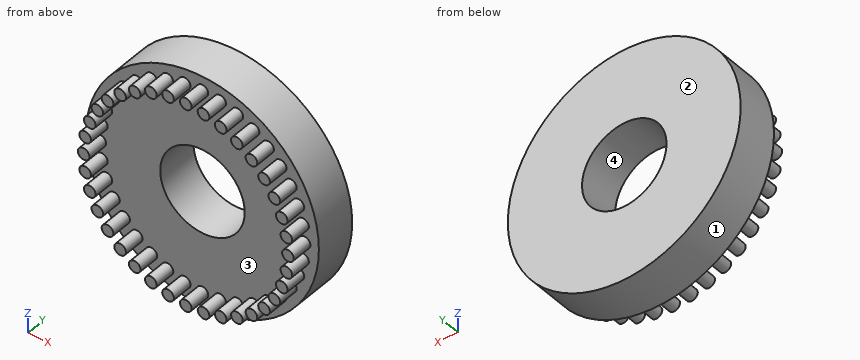
```python
from build123d import *

# Parameters (mm, degrees)
F0_R     = 35
F1_DEPTH = 12.7
F2_R     = 1.75
F3_DEPTH = 6.35
F4_R     = 12.7
F5_DEPTH = 12.701


with BuildPart() as f1:
    # F0 (on Front) → F1 (new body)
    with BuildSketch(Plane.XZ):
        Circle(F0_R)
    extrude(amount=F1_DEPTH)

    # F2 (on face) → F3 (join)
    with BuildSketch(Plane.XZ.offset(12.7)):
        with Locations((-30.708063, 0)):
            Circle(F2_R)
        with Locations((-30.241539, 5.332399)):
            Circle(F2_R)
        with Locations((-28.856141, 10.502776)):
            Circle(F2_R)
        with Locations((-26.593963, 15.354032)):
            Circle(F2_R)
        with Locations((-23.523741, 19.738763)):
            Circle(F2_R)
        with Locations((-19.738763, 23.523741)):
            Circle(F2_R)
        with Locations((-15.354032, 26.593963)):
            Circle(F2_R)
        with Locations((-10.502776, 28.856141)):
            Circle(F2_R)
        with Locations((-5.332399, 30.241539)):
            Circle(F2_R)
        with Locations((0, 30.708063)):
            Circle(F2_R)
        with Locations((5.332399, 30.241539)):
            Circle(F2_R)
        with Locations((10.502776, 28.856141)):
            Circle(F2_R)
        with Locations((15.354032, 26.593963)):
            Circle(F2_R)
        with Locations((19.738763, 23.523741)):
            Circle(F2_R)
        with Locations((23.523741, 19.738763)):
            Circle(F2_R)
        with Locations((26.593963, 15.354032)):
            Circle(F2_R)
        with Locations((28.856141, 10.502776)):
            Circle(F2_R)
        with Locations((30.241539, 5.332399)):
            Circle(F2_R)
        with Locations((30.708063, 0)):
            Circle(F2_R)
        with Locations((30.241539, -5.332399)):
            Circle(F2_R)
        with Locations((28.856141, -10.502776)):
            Circle(F2_R)
        with Locations((26.593963, -15.354032)):
            Circle(F2_R)
        with Locations((23.523741, -19.738763)):
            Circle(F2_R)
        with Locations((19.738763, -23.523741)):
            Circle(F2_R)
        with Locations((15.354032, -26.593963)):
            Circle(F2_R)
        with Locations((10.502776, -28.856141)):
            Circle(F2_R)
        with Locations((5.332399, -30.241539)):
            Circle(F2_R)
        with Locations((0, -30.708063)):
            Circle(F2_R)
        with Locations((-5.332399, -30.241539)):
            Circle(F2_R)
        with Locations((-10.502776, -28.856141)):
            Circle(F2_R)
        with Locations((-15.354032, -26.593963)):
            Circle(F2_R)
        with Locations((-19.738763, -23.523741)):
            Circle(F2_R)
        with Locations((-23.523741, -19.738763)):
            Circle(F2_R)
        with Locations((-26.593963, -15.354032)):
            Circle(F2_R)
        with Locations((-28.856141, -10.502776)):
            Circle(F2_R)
        with Locations((-30.241539, -5.332399)):
            Circle(F2_R)
    extrude(amount=F3_DEPTH)

    # F4 (on face) → F5 (cut, through all)
    with BuildSketch(Plane.XZ.offset(12.7)):
        Circle(F4_R)
    extrude(amount=-F5_DEPTH, mode=Mode.SUBTRACT)


solid = f1.part
```
Design review of the part built by this model. Coordinates are the model's own, in mm. Face numbers are marked on the shaded views. Coordinates: 2 decimals unless noted, no trailing zeros. Order: outer loops, then holes, each group sorted by start corner. A loop starts at its lowest first (then second) coordinate and runs counter-clockwise, first axis right, second up. Notation, with made-up numbers: (-12, -1) - (10, -1) arc R16 cw to (10, 9) - close; hole circle Ø2 at (19.25, -14). An arc over 180 degrees is marked (long way). One line per question, with ' | ' between items.
Q1. To check wall thickness, follow line 1 along Z through (x, y) = (0, -4); line 2 along X through (y, z) = (-10.75, 17); line 3 along Y through (x, z) = (-21, 11.5). State the ranges of each line that lie inside material, in increasing order.
Answer key:
line 1: z = -35 to -12.7, 12.7 to 35 | line 2: x = -30.59 to 30.59 | line 3: y = -12.7 to 0
Q2. The part is to be moulded in two halves that separate along X. For the marked faces 1, 2, 3 and 4, say which applies: +X half, -X half, draft (parallel to the pull), parting line (faces both ways), or undercut.
Answer key:
face 1: parting line | face 2: draft | face 3: undercut | face 4: undercut
Q3. Consider section A-A, the plane z = 0. Give the boundary of the cut face in (x, y).
Answer key:
outline: (-35, -12.7) - (-32.46, -12.7) - (-32.46, -19.05) - (-28.96, -19.05) - (-28.96, -12.7) - (-12.7, -12.7) - (-12.7, 0) - (-35, 0) - close; (12.7, -12.7) - (28.96, -12.7) - (28.96, -19.05) - (32.46, -19.05) - (32.46, -12.7) - (35, -12.7) - (35, 0) - (12.7, 0) - close
Q4. Clearance check with flat-ended pins moving along their axes: pin 1 Ø4 at (x, y) = (-13.5, -17) entering from -Z; pin 2 Ø5 at (y, z) = (-8.5, -23) entering from +X; pin 3 Ø12 at (x, z) = (-2, 16.5) entering from -Y; pin 4 Ø6 at (x, z) = (10.5, -14.5) entering from +Y. State where each tip first meets the part, or that it passes through.
Answer key:
pin 1: stops at z = -30.29 | pin 2: stops at x = 28.37 | pin 3: stops at y = -12.7 | pin 4: stops at y = 0
Q5. Consider section C-C, the plane y = -14.75. Give the number of separate pieces and of enclosed holes in the cut face, then the cut area to 3 significant figures.
Answer key:
separate pieces: 36 | enclosed holes: 0 | area: 346 mm2
Q6. Consider section D-D, the plane x = -19.5. Give the boundary of the cut face in (y, z), then the cut area to 3 significant figures.
Answer key:
outline: (-19.05, -25.26) - (-12.7, -25.26) - (-12.7, -29.06) - (0, -29.06) - (0, 29.06) - (-12.7, 29.06) - (-12.7, 25.26) - (-19.05, 25.26) - (-19.05, 21.79) - (-12.7, 21.79) - (-12.7, -21.79) - (-19.05, -21.79) - close | area: 782 mm2
Q7. Consider section B-B, the plane x = 0. Give the boundary of the cut face in (y, z).
Answer key:
outline: (-19.05, -32.46) - (-12.7, -32.46) - (-12.7, -35) - (0, -35) - (0, -12.7) - (-12.7, -12.7) - (-12.7, -28.96) - (-19.05, -28.96) - close; (-19.05, 28.96) - (-12.7, 28.96) - (-12.7, 12.7) - (0, 12.7) - (0, 35) - (-12.7, 35) - (-12.7, 32.46) - (-19.05, 32.46) - close
